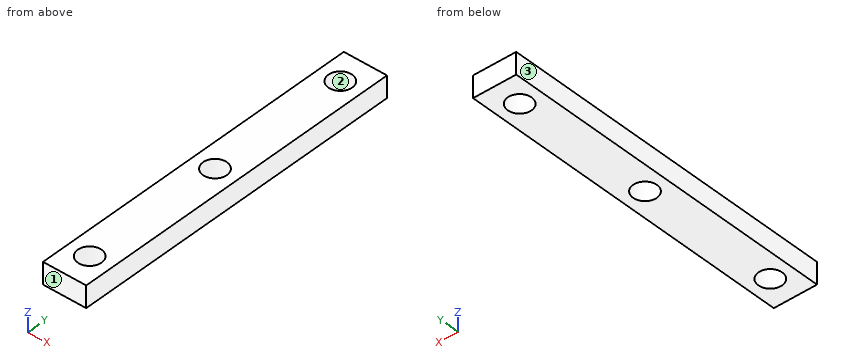
from build123d import *

# Parameters (mm, degrees)
F0_W     = 19.05
F0_H     = 150
F1_DEPTH = 9.525
F2_R     = 5.25
F3_DEPTH = 25.4
F4_R     = 5.25
F5_DEPTH = 25.4


# Not quite as in the source:
# - a length typed as a fraction of an inch, garbled in the dataset ("3 / 203.2 mm" for 3/8 in), is restored


with BuildPart() as f1:
    # F0 (on Top) → F1 (new body)
    with BuildSketch(Plane.XY):
        Rectangle(F0_W, F0_H)
    extrude(amount=F1_DEPTH)

    # F2 (on face) → F3 (cut)
    with BuildSketch(Plane.XY.offset(9.525)):
        with Locations((0, 62.5)):
            Circle(F2_R)
        with Locations((0, -62.5)):
            Circle(F2_R)
    extrude(amount=-F3_DEPTH, mode=Mode.SUBTRACT)

    # F4 (on face) → F5 (cut)
    with BuildSketch(Plane.XY.offset(9.525)):
        Circle(F4_R)
    extrude(amount=-F5_DEPTH, mode=Mode.SUBTRACT)


solid = f1.part
Design review of the part built by this model. Coordinates are the model's own, in mm. Face numbers are marked on the shaded views. Round coordinates to 2 decimals unless told otherwise and drop trailing zeros. Write each loop counter-clockwise with the first axis right and the second up, starting at its lowest first coordinate (ties: lowest second). Pieces come first, ordered by that corner, then holes. Notation, with made-up numbers: M -9.75,-32.5 L 0.25,-32.5 A26 ccw 0.25,-1.5 Z; hole C 68,50 d6. An arc over 180 degrees is marked long. One line per item, written item: value. Start each with the question number.
1. Take a section at A-A on x = 0. State the section outline as (y, z) points (3 decimals).
2. Take a section at D-D on y = -64.5. State the section outline as (x, z) points (3 decimals), then the cut area to 3 significant figures.
3. Clearance check with a flat-ended pin moving along its axis: P1, Ø4, axis at x = -4, y = -46.5, coming from the -Z side. State where the tip first meets the part, or that it passes through.
4. Take a section at C-C on z = 5.75. State the section outline as (x, y) points (3 decimals), then the cut area to 3 significant figures.
5. To check wall thickness, follow probe 1 along Y at (x, z) = (0, 2); probe 2 along Y at (x, z) = (-3.5, 3.25); probe 3 along X at (y, z) = (65, 3) (3 decimals). State the ranges of each line that lie inside material, in increasing order. Write a range as from..to.
6. Take a section at B-B on y = 0. State the section outline as (x, z) points (3 decimals), then the cut area to 3 significant figures.
7. Draft analysis for pull direction Y (two halves, no side actions). For the marked faces 1, 2 and 3, state which applies: pulls with the +Y half, pulls with the -Y half, needs draft (parallel to the pull), parting line crosses it, or undercut.
Computed:
1. outline: M -75,0 L -67.75,0 L -67.75,9.525 L -75,9.525 Z; M -57.25,0 L -5.25,0 L -5.25,9.525 L -57.25,9.525 Z; M 5.25,0 L 57.25,0 L 57.25,9.525 L 5.25,9.525 Z; M 67.75,0 L 75,0 L 75,9.525 L 67.75,9.525 Z
2. outline: M -9.525,0 L -4.854,0 L -4.854,9.525 L -9.525,9.525 Z; M 4.854,0 L 9.525,0 L 9.525,9.525 L 4.854,9.525 Z
2. area: 89.0 mm²
3. P1: stops at z = 0
4. outline: M -9.525,-75 L 9.525,-75 L 9.525,75 L -9.525,75 Z; hole C 0,-62.5 d10.5; hole C 0,0 d10.5; hole C 0,62.5 d10.5
4. area: 2,600 mm²
5. probe 1: y = -75..-67.75, -57.25..-5.25, 5.25..57.25, 67.75..75
5. probe 2: y = -75..-66.41, -58.59..-3.91, 3.91..58.59, 66.41..75
5. probe 3: x = -9.525..-4.617, 4.617..9.525
6. outline: M -9.525,0 L -5.25,0 L -5.25,9.525 L -9.525,9.525 Z; M 5.25,0 L 9.525,0 L 9.525,9.525 L 5.25,9.525 Z
6. area: 81.4 mm²
7. face 1: pulls with the -Y half
7. face 2: undercut
7. face 3: needs draft
